```python
from build123d import *

# Parameters (mm, degrees)
SKETCH1_W           = 52
SKETCH1_H           = 28
BOSS_EXTRUDE1_DEPTH = 1.6
SKETCH2_W           = 18
SKETCH2_H           = 18
BOSS_EXTRUDE2_DEPTH = 3.2
SKETCH3_W           = 3.2
SKETCH3_H           = 8.9
BOSS_EXTRUDE3_DEPTH = 3.2
SKETCH4_W           = 43
SKETCH4_H           = 2.54
BOSS_EXTRUDE4_DEPTH = 5.8


with BuildPart() as part:
    # Sketch1 → Boss-Extrude1 (new body)
    with BuildSketch(Plane(origin=(0, 9, 0), x_dir=(1, 0, 0), z_dir=(0, 1, 0))):
        with Locations((35, 0)):
            Rectangle(SKETCH1_W, SKETCH1_H)
    extrude(amount=BOSS_EXTRUDE1_DEPTH)

    # Sketch2 → Boss-Extrude2 (add)
    with BuildSketch(Plane(origin=(0, 10.6, 0), x_dir=(1, 0, 0), z_dir=(0, 1, 0))):
        with Locations((25, 0)):
            Rectangle(SKETCH2_W, SKETCH2_H)
    extrude(amount=BOSS_EXTRUDE2_DEPTH)

    # Sketch3 → Boss-Extrude3 (add)
    with BuildSketch(Plane(origin=(0, 10.6, 0), x_dir=(1, 0, 0), z_dir=(0, 1, 0))):
        with Locations((60.8, 0)):
            Rectangle(SKETCH3_W, SKETCH3_H)
    extrude(amount=BOSS_EXTRUDE3_DEPTH)

    # Sketch4 → Boss-Extrude4 (add)
    with BuildSketch(Plane(origin=(0, 9, 0), x_dir=(1, 0, 0), z_dir=(0, 1, 0))):
        with Locations((35.5, 11.43)):
            Rectangle(SKETCH4_W, SKETCH4_H)
        with Locations((35.5, -11.43)):
            Rectangle(SKETCH4_W, SKETCH4_H)
    extrude(amount=-BOSS_EXTRUDE4_DEPTH)


solid = part.part
```
Verification items for the finished model (mm, model axes). A direction names the side the tool comes from. Round coordinates to 2 decimals unless told otherwise and drop trailing zeros. Order: outer loops, then holes, each group sorted by start corner. A loop starts at its lowest first (then second) coordinate and runs counter-clockwise, first axis right, second up.
1) Cross-section at C-C, the plane x = 55. Record the cut outline in (y, z), plus the area to 3 significant figures.
Geometry says:
outline: (3.2, -12.7) - (9, -12.7) - (9, -14) - (10.6, -14) - (10.6, 14) - (9, 14) - (9, 12.7) - (3.2, 12.7) - (3.2, 10.16) - (9, 10.16) - (9, -10.16) - (3.2, -10.16) - close
area: 74.3 mm2
2) Cross-section at D-D, the plane y = 7.5. Record the cut outline in (x, z), plus the area to 3 significant figures.
Geometry says:
outline: (14, -12.7) - (57, -12.7) - (57, -10.16) - (14, -10.16) - close; (14, 10.16) - (57, 10.16) - (57, 12.7) - (14, 12.7) - close
area: 218 mm2
3) Cross-section at A-A, the plane y = 12.25. Record the cut outline in (x, z), plus the area to 3 significant figures.
Geometry says:
outline: (16, -9) - (34, -9) - (34, 9) - (16, 9) - close; (59.2, -4.45) - (62.4, -4.45) - (62.4, 4.45) - (59.2, 4.45) - close
area: 352 mm2
4) Depth check by flat-ended pin: pin 1 (3 mm diameter, centred on y = 5.5, z = -11.5, fed in from +X); pin 2 (0.8 mm diameter, centred on y = 6, z = 11.5, fed in from -X); pin 3 (8 mm diameter, centred on x = 34.5, z = 6, fed in from +Y); pin 4 (1.6 mm diameter, centred on x = 61.5, y = 12, fed in from -Z). Enter the tip coordinate at first touch or a pass-through.
Geometry says:
pin 1: stops at x = 57
pin 2: stops at x = 14
pin 3: stops at y = 13.8
pin 4: stops at z = -4.45
5) Draft check along X on faces 5 (the flat face through (35, 6, 12.7)), 6 (the flat face through (34, 12, 0)), 7 (the flat face through (16, 12, 0)). Enter one of: +X half, -X half, draft (parallel to the pull), parting line (faces both ways), or undercut.
Geometry says:
face 5: draft
face 6: undercut
face 7: -X half
6) Tool access check on faces 1 (the flat face through (14, 6, -11)), 2 (the flat face through (61, 10, 0)), 3 (the flat face through (61, 12, 4.45)), 4 (the flat face through (35, 6, -12.7)). Record the directions out of +Z, -Z, +X, -X, +Y, -Y that give a thin tool (end or side, any length) a straight path to the whole face; none if there is none.
Geometry says:
face 1: +Z, -Z, -X, -Y
face 2: +Z, -Z, +X, -Y
face 3: +Z, +X, +Y
face 4: -Z, +X, -X, -Y
7) Material ranges on line 1 (Z direction, x = 40, y = 8.25); line 2 (X direction, y = 12.5, z = -2.25); line 3 (Z direction, x = 60, y = 11.25), recorded low to high.
Geometry says:
line 1: z = -12.7 to -10.16, 10.16 to 12.7
line 2: x = 16 to 34, 59.2 to 62.4
line 3: z = -4.45 to 4.45
8) Cross-section at B-B, the plane z = -11. Record the cut outline in (x, y), plus the area to 3 significant figures.
Geometry says:
outline: (9, 9) - (14, 9) - (14, 3.2) - (57, 3.2) - (57, 9) - (61, 9) - (61, 10.6) - (9, 10.6) - close
area: 333 mm2
